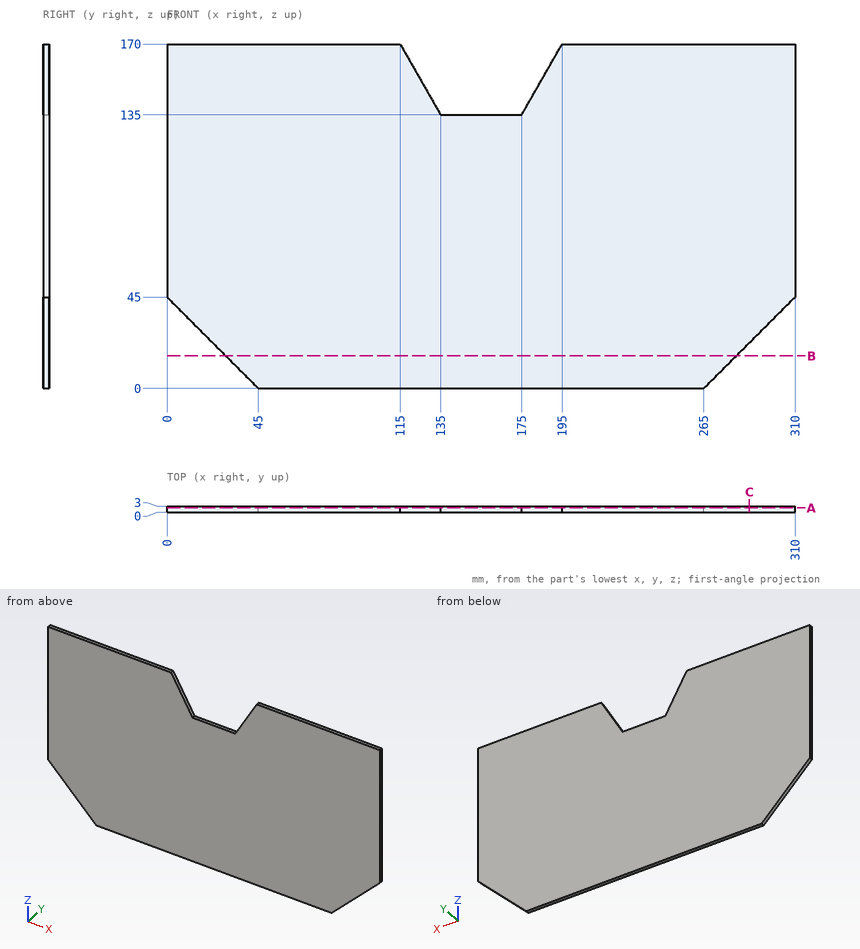
Drawing for the job (mm, zero at the part's lowest x, y, z). Give positions to 0.01 mm unless a question says otherwise; leave off trailing zeros. Loops run counter-clockwise (first coordinate to the right, second up) from the corner with the lowest first, then second, coordinate; pieces in that order, holes last. Notation, with made-up numbers: M 5.5,82 L 51.5,82 A23 cw 51.5,105 Z; hole C 52,78.25 d2. An arc over 180 degrees is marked long. Use one line per item in the form item = value.
Item 1: Flat gauge pin, fed straight in: pin 1 (0.9 mm diameter, centred on x = 158.5, y = 2, fed in from +Z). Where does the tip first touch, or does it go through?
Determined:
pin_1 = 135
Item 2: Drill centre lines: probe 1 along Z at (x, y) = (143.5, 0.8); probe 2 along X at (y, z) = (2.9, 137); probe 3 along X at (y, z) = (2.5, 162). Where is each one in solid material? Low to high. Write a range as from..to.
Determined:
probe_1 = 0..135
probe_2 = 0..133.86, 176.14..310
probe_3 = 0..119.57, 190.43..310
Item 3: Slice it at B-B (z = 16). List the corners of the cut face in (x, y).
Determined:
outline = M 29,0 L 281,0 L 281,3 L 29,3 Z
Item 4: Slice it at A-A (y = 2.25). List the corners of the cut face in (x, z).
Determined:
outline = M 0,45 L 45,0 L 265,0 L 310,45 L 310,170 L 195,170 L 175,135 L 135,135 L 115,170 L 0,170 Z
Item 5: Slice it at C-C (x = 287.5). List the corners of the cut face in (y, z).
Determined:
outline = M 0,22.5 L 3,22.5 L 3,170 L 0,170 Z
